CAD build for the part. Positions are in the model's coordinates, mm. Round coordinates to 2 decimals unless told otherwise and drop trailing zeros. Loops run counter-clockwise (first coordinate to the right, second up) from the corner with the lowest first, then second, coordinate; pieces in that order, holes last.
from build123d import *

# Parameters (mm, degrees)
SKETCH_1_W        = 40
SKETCH_1_H        = 80
EXTRUDE_1_DEPTH   = 2
CHAMFER_1_SIZE    = 2
HOLE_WIZARD_M51_D = 5.5


with BuildPart() as part:
    # Эскиз1 → Бобышка-Вытянуть1 (new body)
    with BuildSketch(Plane(origin=(0, 0, 0), x_dir=(1, 0, 0), z_dir=(0, 1, 0))):
        Rectangle(SKETCH_1_W, SKETCH_1_H)
    extrude(amount=EXTRUDE_1_DEPTH)

    # Фаска1
    chamfer_1_edges = [part.edges().sort_by_distance(p)[0] for p in [
        (20, 1, 40),
        (-20, 1, 40),
        (-20, 1, -40),
        (20, 1, -40),
    ]]
    chamfer(chamfer_1_edges, length=CHAMFER_1_SIZE)

    # Отверстие с зазором M51 (through all)
    with Locations(Plane(origin=(0, 2, 0), x_dir=(1, 0, 0), z_dir=(0, 1, 0))):
        with Locations((-10, 10), (10, 10), (-10, -10), (10, -10), (-10, 30), (10, 30), (10, -30), (-10, -30)):
            Hole(HOLE_WIZARD_M51_D / 2)


solid = part.part
Item 1: Wall check: L1, parallel to X at y = 1.2, z = -10; L2, parallel to Z at x = -10, y = 1.1; L3, parallel to Z at x = -12, y = 0.1. Give the ranges that are in metal, low to high.
Verdict:
L1: x = -20 to -12.75, -7.25 to 7.25, 12.75 to 20
L2: z = -40 to -32.75, -27.25 to -12.75, -7.25 to 7.25, 12.75 to 27.25, 32.75 to 40
L3: z = -40 to -31.89, -28.11 to -11.89, -8.11 to 8.11, 11.89 to 28.11, 31.89 to 40
Item 2: Cut at B-B (x = -10). List the corners of the cut face in (y, z).
Verdict:
outline: (0, -40) - (2, -40) - (2, -32.75) - (0, -32.75) - close; (0, -27.25) - (2, -27.25) - (2, -12.75) - (0, -12.75) - close; (0, -7.25) - (2, -7.25) - (2, 7.25) - (0, 7.25) - close; (0, 12.75) - (2, 12.75) - (2, 27.25) - (0, 27.25) - close; (0, 32.75) - (2, 32.75) - (2, 40) - (0, 40) - close
Item 3: Cut at A-A (y = 0.75). State how many separate pieces and enclosed holes the cut face has, plus the area to 3 significant figures.
Verdict:
separate pieces: 1
enclosed holes: 8
area: 3,000 mm2
Item 4: Mould opens along Z. For faces 1 (the flat face through (0, 1, 40)), 2 (the flat face through (0, 1, -40)), 3 (the cylindrical face through (-12.62, 0.99, 9.17)) say: released by +Z, released by -Z, zero draft, split by the parting line, or undercut.
Verdict:
face 1: released by +Z
face 2: released by -Z
face 3: undercut
Item 5: Flat gauge pin, fed straight in: P1, Ø3.5, axis at x = 10, z = -10, coming from the -Y side. Where does the tip first touch, or does it go through?
Verdict:
P1: passes through
Item 6: Cut at C-C (z = 10). List the corners of the cut face in (x, y).
Verdict:
outline: (-20, 0) - (-12.75, 0) - (-12.75, 2) - (-20, 2) - close; (-7.25, 0) - (7.25, 0) - (7.25, 2) - (-7.25, 2) - close; (12.75, 0) - (20, 0) - (20, 2) - (12.75, 2) - close
